Work out the finished part from the listing and answer in its coordinate system (mm). Face numbers are marked on the shaded views. A direction names the side the tool comes from. Coordinates: 2 decimals unless noted, no trailing zeros. Loops run counter-clockwise (first coordinate to the right, second up) from the corner with the lowest first, then second, coordinate; pieces in that order, holes last. Notation, with made-up numbers: (-2, 16.5) -> (47, 16.5) arc R21 ccw to (47, 45.5) -> close; hole circle Ø7 at (76, 47.5). An arc over 180 degrees is marked (long way). One line per question, with ' | ' between items.
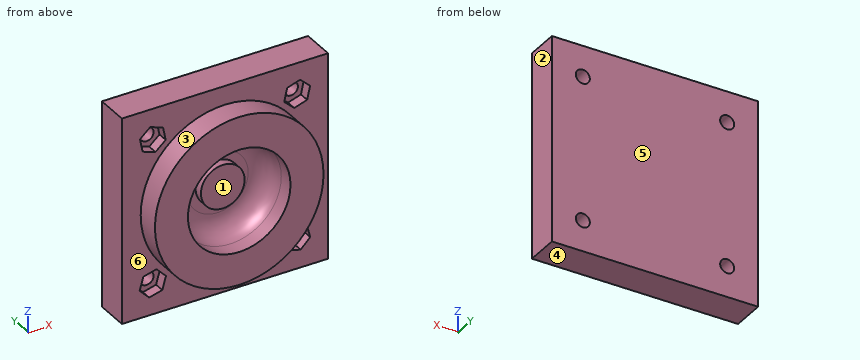
Autodesk Inventor part; units mm, degrees
ref_plane "YZ Plane" through (0, 0, 0) normal (1, 0, 0) x (0, 1, 0)
ref_plane "XZ Plane" through (0, 0, 0) normal (0, 1, 0) x (-1, 0, 0)
ref_plane "XY Plane" through (0, 0, 0) normal (0, 0, 1) x (1, 0, 0)
sketch "Sketch1" plane through (0, 0, 0) normal (0, 0, 1) x (1, 0, 0)
  line L0 (0, -8.6) -> (12.34, -8.6) construction
  line L1 (0, 0) -> (0, -8.6)
  line L2 (0, 0) -> (0, -2.1)
  line L3 (0, -2.1) -> (5.3, -2.1)
  line L4 (5.3, -2.1) -> (5.3, 0)
  line L5 (5.3, 0) -> (7.44, 0)
  line L6 (12.44, -8.7) -> (12.44, -5)
  arc A0 (12.44, -5) -> (7.44, 0) centre (7.44, -5) ccw
  line L7 (12.44, -8.7) -> (20.44, -8.7)
  line L8 (20.44, -8.7) -> (20.44, 5)
  line L9 (20.44, 5) -> (0, 5)
  line L10 (0, 5) -> (0, -2.1)
  line L11 (-4.088, 0) -> (24.528, 0)
  dimension "d2" = 12.34
  dimension "d3" = 8.6
  dimension "d7" = 0
  dimension "d11" = 5.3
  dimension "d12" = 2.1
  dimension "d14" = 5
  dimension "d15" = 8
  dimension "d16" = 13.7
  dimension "d17" = 3.7
  dimension "d18" = 5
revolve "Revolution2" add sketch "Sketch1" angle 360 about axis through (0, 5, 0) along (0, -1, 0)
sketch "Sketch2" plane through (0, 5, 0) normal (0, 1, 0) x (1, 0, 0)
  line L0 (-25, 25) -> (25, 25)
  line L1 (25, 25) -> (25, -25)
  line L2 (25, -25) -> (-25, -25)
  line L3 (-25, -25) -> (-25, 25)
  line L4 (-17.5, 17.5) -> (17.5, 17.5) construction
  line L5 (17.5, 17.5) -> (17.5, -17.5) construction
  line L6 (17.5, -17.5) -> (-17.5, -17.5) construction
  line L7 (-17.5, -17.5) -> (-17.5, 17.5) construction
  circle A0 centre (-17.5, 17.5) radius 1.7
  circle A1 centre (17.5, 17.5) radius 1.7
  circle A2 centre (-17.5, -17.5) radius 1.7
  circle A3 centre (17.5, -17.5) radius 1.7
  line L8 (18.3404, 20.6818) -> (20.6757, 18.3631)
  line L9 (20.6757, 18.3631) -> (19.8353, 15.1813)
  line L10 (19.8353, 15.1813) -> (16.6596, 14.3182)
  line L11 (16.6596, 14.3182) -> (14.3243, 16.6369)
  line L12 (14.3243, 16.6369) -> (15.1647, 19.8187)
  line L13 (15.1647, 19.8187) -> (18.3404, 20.6818)
  line L14 (-16.6058, 14.3329) -> (-19.7956, 15.142)
  line L15 (-19.7956, 15.142) -> (-20.6899, 18.3091)
  line L16 (-20.6899, 18.3091) -> (-18.3942, 20.6671)
  line L17 (-18.3942, 20.6671) -> (-15.2044, 19.858)
  line L18 (-15.2044, 19.858) -> (-14.3101, 16.6909)
  line L19 (-14.3101, 16.6909) -> (-16.6058, 14.3329)
  line L20 (-15.0239, -19.6677) -> (-18.1393, -20.7282)
  line L21 (-18.1393, -20.7282) -> (-20.6153, -18.5605)
  line L22 (-20.6153, -18.5605) -> (-19.9761, -15.3323)
  line L23 (-19.9761, -15.3323) -> (-16.8607, -14.2718)
  line L24 (-16.8607, -14.2718) -> (-14.3847, -16.4395)
  line L25 (-14.3847, -16.4395) -> (-15.0239, -19.6677)
  line L26 (19.9241, -15.2743) -> (20.6396, -18.4864)
  line L27 (20.6396, -18.4864) -> (18.2155, -20.7122)
  line L28 (18.2155, -20.7122) -> (15.0759, -19.7257)
  line L29 (15.0759, -19.7257) -> (14.3604, -16.5136)
  line L30 (14.3604, -16.5136) -> (16.7845, -14.2878)
  line L31 (16.7845, -14.2878) -> (19.9241, -15.2743)
  circle A4 centre (0, 0) radius 12.44
  circle A5 centre (0, 0) radius 12.44
  point P0 (17.5, 17.5)
  dimension "d25" = 35
  dimension "d27" = 17.5
  dimension "d28" = 17.5
  dimension "d29" = 35
  dimension "d30" = 3.4
  dimension "d31" = 3.4
  dimension "d32" = 3.4
  dimension "d33" = 3.4
  dimension "d34" = 5.7
  dimension "d36" = 5.7
  dimension "d37" = 5.7
  dimension "d38" = 5.7
  dimension "d39" = 50
  dimension "d40" = 50
  dimension "d41" = 25
  dimension "d42" = 25
extrude "Extrusion1" add sketch "Sketch2" against normal blind 8 contours L0 L1 L2 L3
extrude "Extrusion2" add sketch "Sketch2" against normal blind 5.5 contours L8 L9 L10 L11 L12 L13 | L14 L15 L16 L17 L18 L19 | L20 L21 L22 L23 L24 L25 | L26 L27 L28 L29 L30 L31
equation "\"d36\" = d34"
equation "\"d37\" = d34"
equation "\"d38\" = d34"
properties part number "BallBearingCupMount"
1) Find the intervals of material crossed by line 1 along X through (y, z) = (3.5, 17.5); line 2 along Y through (x, z) = (21, 1.5), in increasing order.
Check values:
line 1: x = -25 to -19.2, -15.8 to 15.8, 19.2 to 25 | line 2: y = -3 to 5
2) For the marked faces 5 and 6, determine the directions among +Z, -Z, +X, -X, +Y, -Y from which every point of the face is accessible in a straight line to the end or side of a thin tool.
Check values:
face 5: +Z, -Z, +X, -X, +Y | face 6: -Y
3) Find section B-B (x = 0). Write down the section's boundary in (y, z), plus the area to 3 significant figures.
Check values:
outline: (-8.7, -20.44) -> (-3, -20.44) -> (-3, -25) -> (5, -25) -> (5, 25) -> (-3, 25) -> (-3, 20.44) -> (-8.7, 20.44) -> (-8.7, 12.44) -> (-5, 12.44) arc R5 cw to (0, 7.44) -> (0, 5.3) -> (-2.1, 5.3) -> (-2.1, -5.3) -> (0, -5.3) -> (0, -7.44) arc R5 cw to (-5, -12.44) -> (-8.7, -12.44) -> close | area: 450 mm^2
4) Flat-ended cylindrical pins translate along their axes: pin 1 (3 mm diameter, centred on x = 1, z = -1.5, fed in from -Y); pin 2 (5 mm diameter, centred on x = -16, z = 19, fed in from -Y); pin 3 (2 mm diameter, centred on y = -6, z = -1.5, fed in from -X); pin 4 (4 mm diameter, centred on x = 17.5, z = -17.5, fed in from +Y). Find the tip coordinate at first contact, or state that the pin passes through.
Check values:
pin 1: stops at y = -2.1 | pin 2: stops at y = -3 | pin 3: stops at x = -20.43 | pin 4: stops at y = 5
5) Find section A-A (z = 17.5). Write down the section's boundary in (x, y).
Check values:
outline: (-25, -3) -> (-20.41, -3) -> (-20.41, -0.5) -> (-19.2, -0.5) -> (-19.2, 5) -> (-25, 5) -> close; (-15.8, -0.5) -> (-14.59, -0.5) -> (-14.59, -3) -> (-10.56, -3) -> (-10.56, -8.7) -> (10.56, -8.7) -> (10.56, -3) -> (14.58, -3) -> (14.58, -0.5) -> (15.8, -0.5) -> (15.8, 5) -> (-15.8, 5) -> close; (19.2, -0.5) -> (20.42, -0.5) -> (20.42, -3) -> (25, -3) -> (25, 5) -> (19.2, 5) -> close
6) Find section C-C (z = 0). Write down the section's boundary in (x, y).
Check values:
outline: (-25, -3) -> (-20.44, -3) -> (-20.44, -8.7) -> (-12.44, -8.7) -> (-12.44, -5) arc R5 cw to (-7.44, 0) -> (-5.3, 0) -> (-5.3, -2.1) -> (5.3, -2.1) -> (5.3, 0) -> (7.44, 0) arc R5 cw to (12.44, -5) -> (12.44, -8.7) -> (20.44, -8.7) -> (20.44, -3) -> (25, -3) -> (25, 5) -> (-25, 5) -> close
7) The mould has two halves that part along Z. Classify the marked faces 1, 2, 3 and 4: released by +Z, released by -Z, zero draft, split by the parting line, or undercut.
Check values:
face 1: undercut | face 2: zero draft | face 3: split by the parting line | face 4: released by -Z
8) Find section D-D (y = -6.5). Write down the section's boundary in (x, z), plus the area to 3 significant figures.
Check values:
outline: circle Ø40.88 at (0, 0); hole circle Ø24.88 at (0, 0) | area: 826 mm^2
